For this review, take the finished solid that the model builds, in its own axes (mm). Coordinates: 2 decimals unless noted, no trailing zeros. Write each loop counter-clockwise with the first axis right and the second up, starting at its lowest first coordinate (ties: lowest second). Pieces come first, ordered by that corner, then holes. Notation, with made-up numbers: (-13.5, 77) -> (-3.5, 77) arc R13 cw to (-3.5, 100) -> close; hole circle Ø4 at (-29.75, -38). An arc over 180 degrees is marked (long way). One line per item, written item: value. Start each with the question number.
1) Add section B-B (y = 116). State the section outline as (x, z) points.
2) Add section A-A (z = -511). State the section outline as (x, y) points, and give its area (3 significant figures).
3) For pin 1 Ø2 at (x, y) = (-5, 96) entering from +Z; pin 2 Ø4.5 at (x, y) = (-5, -12.5) entering from -Z; pin 3 Ø3 at (x, z) = (-2.5, -535) entering from -Y, all flat-tipped, find the tip position at first contact; note any pin that passes through.
4) For probe 1 along Y at (x, z) = (-5.75, -135.5); probe 2 along Y at (x, z) = (-6.75, -247.5); probe 3 along Z at (x, y) = (-3.75, 108.5), list the stretches that pass through material, from the lowest coordinate up. Write a range as from..to.
from build123d import *

# Parameters (mm, degrees)
BASE_FLANGE1_DEPTH = 8
FILLET_1_0_R       = 1


# Sheet-metal steps are written as plain solids
with BuildPart() as part:
    # Sketch1 → Base-Flange1 (new body)
    with BuildSketch(Plane(origin=(0, 0, 0), x_dir=(0, 0, -1), z_dir=(1, 0, 0))):
        with BuildLine():
            Line((531, -15), (442.5, -15))
            Line((442.5, -15), (442.5, -9))
            Line((442.5, -9), (354, -9))
            Line((354, -9), (354, -15))
            Line((354, -15), (265.5, -15))
            Line((265.5, -15), (265.5, -9))
            Line((265.5, -9), (177, -9))
            Line((177, -9), (177, -15))
            Line((177, -15), (88.5, -15))
            Line((88.5, -15), (88.5, -9))
            Line((88.5, -9), (0, -9))
            Line((0, -9), (0, 10))
            Line((0, 10), (17.311064102, 31))
            Line((17.311064102, 31), (527.748052756, 31))
            ThreePointArc((527.748052756, 31), (697.748052756, 89.840336788), (795, 241.181818182))
            Line((795, 241.181818182), (839.703962084, 230.339504132))
            ThreePointArc((839.703962084, 230.339504132), (826.746837948, 189.2327939), (808.257153356, 150.299771211))
            Line((808.257153356, 150.299771211), (813.503193561, 147.387888287))
            ThreePointArc((813.503193561, 147.387888287), (789.433768579, 110.742928998), (760.560188707, 77.750404912))
            Line((760.560188707, 77.750404912), (756.275511236, 81.951113323))
            ThreePointArc((756.275511236, 81.951113323), (726.159050553, 55.606079515), (692.923211747, 33.325122864))
            Line((692.923211747, 33.325122864), (695.938293543, 28.137816444))
            ThreePointArc((695.938293543, 28.137816444), (654.250802879, 7.812798402), (610.053579846, -6.242759659))
            Line((610.053579846, -6.242759659), (608.523872748, -0.439504608))
            ThreePointArc((608.523872748, -0.439504608), (572.452930854, -6.852497602), (535.879339812, -9))
            Line((535.879339812, -9), (531, -9))
            Line((531, -9), (531, -15))
        make_face()
    extrude(amount=-BASE_FLANGE1_DEPTH)

    # Fillet-1.0
    fillet_1_0_edges = [part.edges().sort_by_distance(p)[0] for p in [
        (-4, 31, -17.311064102),
        (-4, 241.181818182, -795),
        (-4, 230.339504132, -839.703962084),
        (-4, 150.299771211, -808.257153356),
        (-4, 147.387888287, -813.503193561),
        (-4, 77.750404912, -760.560188707),
        (-4, 81.951113323, -756.275511236),
        (-4, 33.325122864, -692.923211747),
        (-4, 28.137816444, -695.938293543),
        (-4, -6.242759659, -610.053579846),
        (-4, -0.439504608, -608.523872748),
        (-4, -9, -531),
        (-4, -15, -531),
        (-4, -15, -442.5),
        (-4, -9, -442.5),
        (-4, -9, -354),
        (-4, -15, -354),
        (-4, -15, -265.5),
        (-4, -9, -265.5),
        (-4, -9, -177),
        (-4, -15, -177),
        (-4, -15, -88.5),
        (-4, -9, -88.5),
        (-4, -9, 0),
    ]]
    fillet(fillet_1_0_edges, radius=FILLET_1_0_R)


solid = part.part
Numbers:
1. outline: (-8, -793.35) -> (0, -793.35) -> (0, -726.56) -> (-8, -726.56) -> close
2. outline: (-8, -15) -> (0, -15) -> (0, 31) -> (-8, 31) -> close
2. area: 368 mm²
3. pin 1: z = -704.11
3. pin 2: z = -531
3. pin 3: y = -9
4. probe 1: -15..31
4. probe 2: -9..31
4. probe 3: -787.71..-719.11
